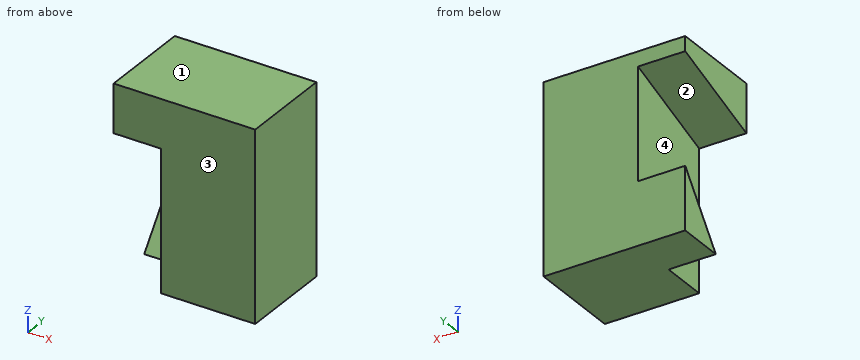
```python
from build123d import *

# Parameters (mm, degrees)
F0_W     = 38.1
F0_H     = 50.8
F1_DEPTH = 25.4
F3_DEPTH = 12.7


# Not quite as in the source:
# - a length typed as a fraction of an inch, garbled in the dataset ("3 / 203.2 mm" for 3/8 in), is restored


with BuildPart() as f1:
    # F0 (on Front) → F1 (new body)
    with BuildSketch(Plane.XZ):
        with Locations((19.05, 25.4)):
            Rectangle(F0_W, F0_H)
    extrude(amount=F1_DEPTH)

    # F2 (on face) → F3 (cut)
    with BuildSketch(Plane(origin=(0, 0, 0), x_dir=(0, -1, 0), z_dir=(-1, 0, 0))):
        Polygon((25.4, 0), (25.4, 37.7936698496), (0, 46.8400232494), (0, 16.886530444), (12.7, 0), align=None)
    extrude(amount=-F3_DEPTH, mode=Mode.SUBTRACT)


solid = f1.part
```
Build history of the part. All positions in model axes, mm. Face numbers are marked on the shaded views. Give positions to 0.01 mm unless a question says otherwise; leave off trailing zeros. Order: outer loops, then holes, each group sorted by start corner. A loop starts at its lowest first (then second) coordinate and runs counter-clockwise, first axis right, second up. Notation, with made-up numbers: M 74.5,-8 L 104.5,-8 A28 cw 104.5,16 Z; hole C 23,-16 d9. An arc over 180 degrees is marked long. Return JSON: item names as keys, results as strings.
Q1. Band-saw the part on D-D (y = -11.75). Give the cut face in (x, z).
Answer list:
{"outline": "M 0,0 L 38.1,0 L 38.1,50.8 L 0,50.8 L 0,42.66 L 12.7,42.66 L 12.7,1.26 L 0,1.26 Z"}
Q2. Band-saw the part on B-B (y = -8.5). Give the cut face in (x, z), then the cut area to 3 significant figures.
Answer list:
{"outline": "M 0,0 L 38.1,0 L 38.1,50.8 L 0,50.8 L 0,43.81 L 12.7,43.81 L 12.7,5.58 L 0,5.58 Z", "area": "1,450 mm^2"}
Q3. Flat gauge pin, fed straight in: pin 1 (10 mm diameter, centred on y = -19.5, z = 27.5, fed in from -X). Where does the tip first touch, or does it go through?
Answer list:
{"pin 1": "stops at x = 12.7"}
Q4. Two-plate mould, pull along Z, no slides. Class the marked faces 1, 2, 3 and 4: pulls with the +Z half, pulls with the -Z half, needs draft (parallel to the pull), parting line crosses it, or undercut.
Answer list:
{"face 1": "pulls with the +Z half", "face 2": "undercut", "face 3": "needs draft", "face 4": "undercut"}
Q5. Wall check: probe 1 along X at (y, z) = (-3.5, 36); probe 2 along Z at (x, y) = (8, -7); probe 3 along Z at (x, y) = (5, -12.5). Give the ranges that are in metal, low to high. Write a range as from..to.
Answer list:
{"probe 1": "x = 12.7..38.1", "probe 2": "z = 0..7.58, 44.35..50.8", "probe 3": "z = 0..0.27, 42.39..50.8"}
Q6. Band-saw the part on A-A (x = 9). Give the cut face in (y, z), then the cut area to 3 significant figures.
Answer list:
{"outline": "M -25.4,37.79 L 0,46.84 L 0,50.8 L -25.4,50.8 Z; M -12.7,0 L 0,0 L 0,16.89 Z", "area": "323 mm^2"}
Q7. Band-saw the part on C-C (z = 12.5). Give the cut face in (x, y).
Answer list:
{"outline": "M 0,-3.3 L 12.7,-3.3 L 12.7,-25.4 L 38.1,-25.4 L 38.1,0 L 0,0 Z"}
